```python
from build123d import *

# Parameters (mm, degrees)
SKETCH_1_W                 = 240
SKETCH_1_H                 = 146
SKETCH_1_R                 = 3
SKETCH_1_R_2               = 18
SKETCH_1_R_3               = 3.5
EXTRUDE_1_DEPTH            = 2
HOLE_WIZARD_M21_AT_2_COUNT = 2
HOLE_WIZARD_M21_AT_2_PITCH = 224
HOLE_WIZARD_M21_AT_3_COUNT = 2
HOLE_WIZARD_M21_AT_3_PITCH = 258.99034731
HOLE_WIZARD_M21_AT_4_COUNT = 2
HOLE_WIZARD_M21_AT_4_PITCH = 130


with BuildPart() as part:
    # Эскиз1 → Бобышка-Вытянуть1 (new body)
    with BuildSketch(Plane.XY):
        with Locations((120, 73)):
            Rectangle(SKETCH_1_W, SKETCH_1_H)
        with Locations((48.515350749, 26)):
            Circle(SKETCH_1_R, mode=Mode.SUBTRACT)
        with Locations((40, 68.913299822)):
            Circle(SKETCH_1_R, mode=Mode.SUBTRACT)
        with Locations((90.832011317, 93)):
            Circle(SKETCH_1_R, mode=Mode.SUBTRACT)
        with Locations((167, 73)):
            Circle(SKETCH_1_R_2, mode=Mode.SUBTRACT)
        with Locations((20, 138)):
            Circle(SKETCH_1_R_3, mode=Mode.SUBTRACT)
        with Locations((20, 8)):
            Circle(SKETCH_1_R_3, mode=Mode.SUBTRACT)
        with Locations((220, 8)):
            Circle(SKETCH_1_R_3, mode=Mode.SUBTRACT)
        with Locations((220, 138)):
            Circle(SKETCH_1_R_3, mode=Mode.SUBTRACT)
    extrude(amount=EXTRUDE_1_DEPTH)

    # Эскиз5 → Зенковка для винта с полупотайной головкой M21 (revolve, cut)
    with BuildSketch(Plane(origin=(232, 138, 0), x_dir=(0, 1, 0), z_dir=(1, 0, 0))):
        Polygon((0, 0), (0, 2), (1.2, 2), (1.2, 1), (2.2, 0), align=None)
    hole_wizard_m21 = revolve(axis=Axis((232, 138, -6.35), (0, 0, 1)), mode=Mode.SUBTRACT)

    # Зенковка для винта с полупотайной головкой M21 at 2: Зенковка для винта с полупотайной головкой M21 ×2
    with Locations(*[(-i * HOLE_WIZARD_M21_AT_2_PITCH, 0, 0) for i in range(1, HOLE_WIZARD_M21_AT_2_COUNT)]):
        add(hole_wizard_m21, mode=Mode.SUBTRACT)

    # Зенковка для винта с полупотайной головкой M21 at 3: Зенковка для винта с полупотайной головкой M21 ×2
    with Locations(*[Vector(-0.864897099, -0.501949209, 0) * (i * HOLE_WIZARD_M21_AT_3_PITCH) for i in range(1, HOLE_WIZARD_M21_AT_3_COUNT)]):
        add(hole_wizard_m21, mode=Mode.SUBTRACT)

    # Зенковка для винта с полупотайной головкой M21 at 4: Зенковка для винта с полупотайной головкой M21 ×2
    with Locations(*[(0, -i * HOLE_WIZARD_M21_AT_4_PITCH, 0) for i in range(1, HOLE_WIZARD_M21_AT_4_COUNT)]):
        add(hole_wizard_m21, mode=Mode.SUBTRACT)


solid = part.part
```
Here's how the part is built. I have some questions about the finished solid (model axes, mm). Coordinates: 2 decimals unless noted, no trailing zeros. Order: outer loops, then holes, each group sorted by start corner. A loop starts at its lowest first (then second) coordinate and runs counter-clockwise, first axis right, second up. Notation, with made-up numbers: M -19.75,30.25 L 27.25,30.25 A22 cw 27.25,43.25 Z; hole C 67.5,42 d6. An arc over 180 degrees is marked long. Answer as a JSON object with one key per item and string values. Group by question number.
(1) Suppose I cut it at A-A, the plane x = 40. Please give me the cut outline in (y, z).
(2) Suppose I cut it at B-B, the plane x = 221. Please give me the cut outline in (y, z), then the cut area to 3 significant figures.
(3) For pin 1 (1.9 mm diameter, centred on x = 232, y = 8, fed in from -Z); pin 2 (3 mm diameter, centred on x = 232, y = 138, fed in from -Z), each with a flat end and sliding along its axis, tell me the tip position at first contact or that it passes through.
(4) Suppose I cut it at D-D, the plane x = 167. Please give me the cut outline in (y, z), then the cut area to 3 significant figures.
(5) I need wall thicknesses on probe 1 along X at (y, z) = (138, 1.5); probe 2 along Y at (x, z) = (220, 0.7); probe 3 along Y at (x, z) = (8, 1.45). Which ranges of each line are inside material? Lowest first, please.
(6) Suppose I cut it at C-C, the plane z = 1.3. State how many separate pieces and enclosed holes the cut face has, then the cut area to 3 significant figures.
(7) If we mould it in two halves opening along Y, with no side actions, what happens to faces 1 (the face through (118, 74, 2)), 2 (the face through (51.377, 26.901, 0.986))? For each: released by +Y, released by -Y, zero draft, split by the parting line, or undercut.
Values found:
{
 "1": {"outline": "M 0,0 L 65.91,0 L 65.91,2 L 0,2 Z; M 71.91,0 L 146,0 L 146,2 L 71.91,2 Z"},
 "2": {"outline": "M 0,0 L 4.65,0 L 4.65,2 L 0,2 Z; M 11.35,0 L 134.65,0 L 134.65,2 L 11.35,2 Z; M 141.35,0 L 146,0 L 146,2 L 141.35,2 Z", "area": "265 mm^2"},
 "3": {"pin 1": "passes through", "pin 2": "stops at z = 0.7"},
 "4": {"outline": "M 0,0 L 55,0 L 55,2 L 0,2 Z; M 91,0 L 146,0 L 146,2 L 91,2 Z", "area": "220 mm^2"},
 "5": {"probe 1": "x = 0 to 6.8, 9.2 to 16.5, 23.5 to 216.5, 223.5 to 230.8, 233.2 to 240", "probe 2": "y = 0 to 4.5, 11.5 to 134.5, 141.5 to 146", "probe 3": "y = 0 to 6.8, 9.2 to 136.8, 139.2 to 146"},
 "6": {"separate pieces": "1", "enclosed holes": "12", "area": "33,800 mm^2"},
 "7": {"face 1": "zero draft", "face 2": "undercut"}
}
